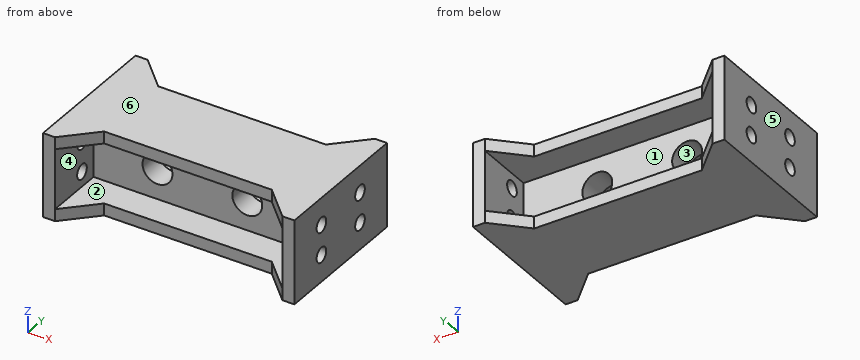
```python
from build123d import *

# Parameters (mm, degrees)
SKETCH2_W               = 42
SKETCH2_H               = 14
BOSS_EXTRUDE1_DEPTH     = 4
SKETCH3_W               = 2
SKETCH3_H               = 14
BOSS_EXTRUDE2_DEPTH     = 10
BOSS_EXTRUDE3_DEPTH     = 2
SKETCH5_R               = 2.5
CUT_EXTRUDE1_DEPTH      = 11
CUT_EXTRUDE1_DEPTH_BACK = 5
SKETCH6_R               = 1.25
CUT_EXTRUDE2_DEPTH      = 2
SKETCH7_W               = 2
SKETCH7_H               = 14
BOSS_EXTRUDE4_DEPTH     = 10
SKETCH8_R               = 1.25
CUT_EXTRUDE3_DEPTH      = 10
BOSS_EXTRUDE5_DEPTH     = 2


with BuildPart() as part:
    # Sketch2 → Boss-Extrude1 (new body)
    with BuildSketch(Plane(origin=(0, 0, 0), x_dir=(1, 0, 0), z_dir=(0, 1, 0))):
        Rectangle(SKETCH2_W, SKETCH2_H)
    extrude(amount=BOSS_EXTRUDE1_DEPTH)

    # Sketch3 → Boss-Extrude2 (add)
    with BuildSketch(Plane.XZ):
        with Locations((-20, 0)):
            Rectangle(SKETCH3_W, SKETCH3_H)
        with Locations((20, 0)):
            Rectangle(SKETCH3_W, SKETCH3_H)
    extrude(amount=BOSS_EXTRUDE2_DEPTH)

    # Sketch4 → Boss-Extrude3 (add)
    with BuildSketch(Plane.XY.offset(7)):
        Polygon((-14, -5), (14, -5), (19, -10), (19, 0), (-19, 0), (-19, -10), align=None)
    boss_extrude3 = extrude(amount=-BOSS_EXTRUDE3_DEPTH)

    # Mirror1: Boss-Extrude3 across plane
    add(boss_extrude3.mirror(Plane.XY))

    # Sketch5 → Cut-Extrude1 (cut, two sides)
    with BuildSketch(Plane.XZ) as cut_extrude1_sk:
        with Locations((-8.319906625, 0)):
            Circle(SKETCH5_R)
        with Locations((6.680093375, 0)):
            Circle(SKETCH5_R)
    extrude(amount=CUT_EXTRUDE1_DEPTH, mode=Mode.SUBTRACT)
    extrude(cut_extrude1_sk.sketch, amount=-CUT_EXTRUDE1_DEPTH_BACK, mode=Mode.SUBTRACT)

    # Sketch6 → Cut-Extrude2 (cut)
    with BuildSketch(Plane(origin=(-19, 0, 0), x_dir=(0, 0, -1), z_dir=(1, 0, 0))):
        with Locations((-2.5, -3)):
            Circle(SKETCH6_R)
        with Locations((2.5, -3)):
            Circle(SKETCH6_R)
    cut_extrude2 = extrude(amount=-CUT_EXTRUDE2_DEPTH, mode=Mode.SUBTRACT)

    # Mirror2: Cut-Extrude2 across plane
    add(cut_extrude2.mirror(Plane(origin=(0, 0, 0), x_dir=(0, 0, 1), z_dir=(1, 0, 0))), mode=Mode.SUBTRACT)

    # Sketch7 → Boss-Extrude4 (add)
    with BuildSketch(Plane(origin=(0, 4, 0), x_dir=(1, 0, 0), z_dir=(0, 1, 0))):
        with Locations((-20, 0)):
            Rectangle(SKETCH7_W, SKETCH7_H)
        with Locations((20, 0)):
            Rectangle(SKETCH7_W, SKETCH7_H)
    extrude(amount=BOSS_EXTRUDE4_DEPTH)

    # Sketch8 → Cut-Extrude3 (cut)
    with BuildSketch(Plane(origin=(-19, 0, 0), x_dir=(0, 0, -1), z_dir=(1, 0, 0))):
        with Locations((-2.5, 7)):
            Circle(SKETCH8_R)
        with Locations((2.5, 7)):
            Circle(SKETCH8_R)
    cut_extrude3 = extrude(amount=-CUT_EXTRUDE3_DEPTH, mode=Mode.SUBTRACT)

    # Mirror3: Cut-Extrude3 across plane
    add(cut_extrude3.mirror(Plane(origin=(0, 0, 0), x_dir=(0, 0, 1), z_dir=(1, 0, 0))), mode=Mode.SUBTRACT)

    # Sketch9 → Boss-Extrude5 (add)
    with BuildSketch(Plane(origin=(0, 0, -7), x_dir=(-1, 0, 0), z_dir=(0, 0, -1))):
        Polygon((19, 14), (19, 4), (-19, 4), (-19, 14), (-14, 9), (14, 9), align=None)
    boss_extrude5 = extrude(amount=-BOSS_EXTRUDE5_DEPTH)

    # Mirror4: Boss-Extrude5 across plane
    add(boss_extrude5.mirror(Plane.XY))


solid = part.part
```
The listing builds one solid part. Answer for the finished solid, in the listing's coordinates (mm). Face numbers are marked on the shaded views. A direction names the side the tool comes from. Coordinates: 2 decimals unless noted, no trailing zeros. Loops run counter-clockwise (first coordinate to the right, second up) from the corner with the lowest first, then second, coordinate; pieces in that order, holes last. Notation, with made-up numbers: M 82.5,1.5 L 113.5,1.5 A26 ccw 113.5,29.5 Z; hole C 17,-13 d3. An arc over 180 degrees is marked long. Answer as a JSON object with one key per item and string values. Group by question number.
Item 1: Each of these flat-tipped pins is pushed along its axis until it touches: P1, Ø3, axis at y = -3, z = 2.5, coming from the +X side; P2, Ø2, axis at x = -3, z = 5.5, coming from the +Y side; P3, Ø8, axis at x = -7, z = -5, coming from the -Y side; P4, Ø8, axis at x = -8.32, z = 0, coming from the -Y side. Where does it stop, or does it pass through?
Item 2: Consider L1, parallel to Y at x = -20.15, z = 2.5; L2, parallel to Z at x = 19.55, y = 7; L3, parallel to Z at x = 4, y = -4.5. Determine where each line is inside the solid, lowest interval first.
Item 3: Section A-A (y = 7) is taken. Write down the section's boundary in (x, z), and give its area (3 significant figures).
Item 4: Section C-C (z = 0) is taken. Write down the section's boundary in (x, y).
Item 5: Which of the six approach directions +Z, -Z, +X, -X, +Y, -Y give full straight-line access (tool end or side, diameter ignored) to the marked faces 1, 2 and 3?
Item 6: Section B-B (z = 6.25) is taken. Write down the section's boundary in (x, y), and give its area (3 significant figures).
Item 7: Determine the mould class of the marked faces 4, 5 and 6 for opening direction Z: +Z half, -Z half, draft (parallel to the pull), parting line (faces both ways), or undercut.
Item 8: Section D-D (x = 15) is taken. Write down the section's boundary in (y, z).
Solved:
{
 "1": {"P1": "stops at x = 21", "P2": "stops at y = 9", "P3": "stops at y = -5", "P4": "stops at y = 0"},
 "2": {"L1": "y = -10 to -4.25, -1.75 to 5.75, 8.25 to 14", "L2": "z = -7 to -3.75, -1.25 to 1.25, 3.75 to 7", "L3": "z = -7 to -5, 5 to 7"},
 "3": {"outline": "M -21,-7 L 21,-7 L 21,-3.75 L 19,-3.75 L 19,-5 L -19,-5 L -19,-3.75 L -21,-3.75 Z; M -21,-1.25 L -19,-1.25 L -19,1.25 L -21,1.25 Z; M -21,3.75 L -19,3.75 L -19,5 L 19,5 L 19,3.75 L 21,3.75 L 21,7 L -21,7 Z; M 19,-1.25 L 21,-1.25 L 21,1.25 L 19,1.25 Z", "area": "188 mm2"},
 "4": {"outline": "M -21,-10 L -19,-10 L -19,0 L -10.82,0 L -10.82,4 L -19,4 L -19,14 L -21,14 Z; M -5.82,0 L 4.18,0 L 4.18,4 L -5.82,4 Z; M 9.18,0 L 19,0 L 19,-10 L 21,-10 L 21,14 L 19,14 L 19,4 L 9.18,4 Z"},
 "5": {"face 1": "+Y", "face 2": "-Y", "face 3": "+Y, -Y"},
 "6": {"outline": "M -21,-10 L -19,-10 L -14,-5 L 14,-5 L 19,-10 L 21,-10 L 21,14 L 19,14 L 14,9 L -14,9 L -19,14 L -21,14 Z", "area": "678 mm2"},
 "7": {"face 4": "undercut", "face 5": "draft", "face 6": "+Z half"},
 "8": {"outline": "M -6,-7 L 10,-7 L 10,-5 L 4,-5 L 4,5 L 10,5 L 10,7 L -6,7 L -6,5 L 0,5 L 0,-5 L -6,-5 Z"}
}
